The drawing under review shows one solid part. Ordinate dimensions are in mm from its lowest x, y, z. A direction names the side the tool comes from. Coordinates: 2 decimals unless noted, no trailing zeros. Write each loop counter-clockwise with the first axis right and the second up, starting at its lowest first coordinate (ties: lowest second). Pieces come first, ordered by that corner, then holes.
Q1. Add section B-B, the plane y = 50. Give the boundary of the cut face in (x, z), plus the area to 3 significant figures.
Q2. Clearance check with flat-ended pins moving along their axes: pin 1 Ø1.5 at (y, z) = (80.5, 1.5) entering from -X; pin 2 Ø1.5 at (y, z) = (47, 2.5) entering from -X; pin 3 Ø2.5 at (x, z) = (17.5, 3.5) entering from +Y. State where each tip first meets the part, or that it passes through.
Q3. To check wall thickness, follow probe 1 along Y at (x, z) = (17.75, 0.55) (1 decimal); probe 2 along Y at (x, z) = (6.5, 4.05); probe 3 along X at (y, z) = (59.5, 1.85). State the ranges of each line that lie inside material, in increasing order.
Q4. Add section A-A, the plane x = 4.25. Give the boundary of the cut face in (y, z) (1 decimal), plus the area to 3 significant figures.
Q5. The part is to be moulded in two halves that separate along Y. For the marked faces 1, 2, 3 and 4, say which applies: +Y half, -Y half, draft (parallel to the pull), parting line (faces both ways), or undercut.
Q6. Machinability: for the marked faces 5, 6 and 7, which of the approach directions +Z, -Z, +X, -X, +Y, -Y give a long, thin tool a straight path to every point of the face, cutting with its end or side? Answer none if there is none.
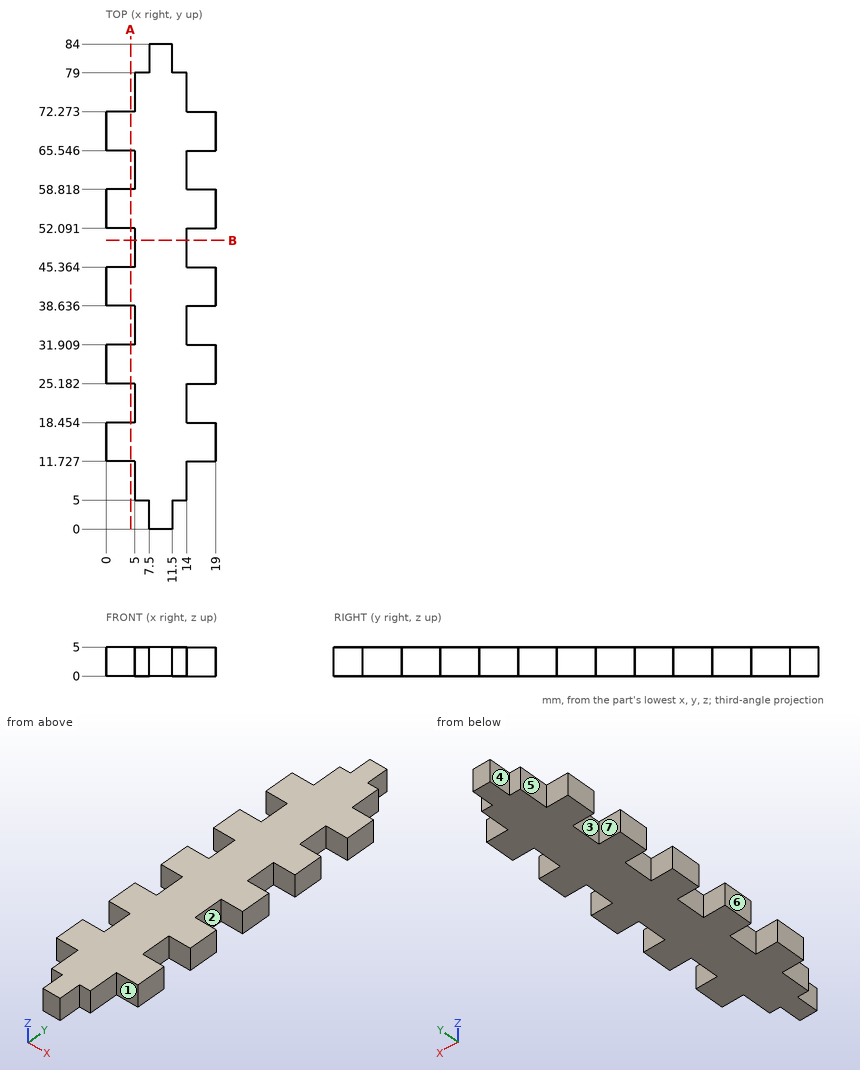
Here are the results:
1. outline: (5, 0) - (14, 0) - (14, 5) - (5, 5) - close
1. area: 45.0 mm2
2. pin 1: stops at x = 7.5
2. pin 2: stops at x = 5
2. pin 3: stops at y = 72.27
3. probe 1: y = 11.7 to 18.5, 25.2 to 31.9, 38.6 to 45.4, 52.1 to 58.8, 65.5 to 72.3
3. probe 2: y = 5 to 79
3. probe 3: x = 5 to 14
4. outline: (11.7, 0) - (18.5, 0) - (18.5, 5) - (11.7, 5) - close; (25.2, 0) - (31.9, 0) - (31.9, 5) - (25.2, 5) - close; (38.6, 0) - (45.4, 0) - (45.4, 5) - (38.6, 5) - close; (52.1, 0) - (58.8, 0) - (58.8, 5) - (52.1, 5) - close; (65.5, 0) - (72.3, 0) - (72.3, 5) - (65.5, 5) - close
4. area: 168 mm2
5. face 1: -Y half
5. face 2: undercut
5. face 3: undercut
5. face 4: draft
6. face 5: +Z, -Z, -X, +Y
6. face 6: +Z, -Z, -X, +Y, -Y
6. face 7: +Z, -Z, -X
